The listing builds one solid part. Answer for the finished solid, in the listing's coordinates (mm). A direction names the side the tool comes from. Round coordinates to 2 decimals unless told otherwise and drop trailing zeros. Write each loop counter-clockwise with the first axis right and the second up, starting at its lowest first coordinate (ties: lowest second). Pieces come first, ordered by that corner, then holes. Notation, with made-up numbers: M -16,34 L 22,34 A14 ccw 22,46 Z; hole C 65,16.25 d1. An arc over 180 degrees is marked long. Answer as CSV lines item,"result". Start each with the question number.
from build123d import *

# Parameters (mm, degrees)
SKETCH_1_R               = 70
EXTRUDE_1_DEPTH          = 12
SKETCH_2_R               = 20
EXTRUDE_2_DEPTH          = 12
SKETCH_3_R               = 8
CUT_EXTRUDE_1_DEPTH      = 102.862652626
CUT_EXTRUDE_2_DEPTH      = 102.862652626
PATTERN_CIRCULAR_1_COUNT = 6
SKETCH_5_R               = 32
CUT_EXTRUDE_3_DEPTH      = 141
PATTERN_CIRCULAR_2_COUNT = 6
SKETCH_6_R               = 4
CUT_EXTRUDE_4_DEPTH      = 140.642
SKETCH_8_R               = 2.5
CUT_EXTRUDE_7_DEPTH      = 13


with BuildPart() as part:
    # Sketch 1 → Extrude 1 (new body)
    with BuildSketch(Plane.XY):
        Circle(SKETCH_1_R)
    extrude(amount=EXTRUDE_1_DEPTH)

    # Sketch 2 → Extrude 2 (add)
    with BuildSketch(Plane.XY.offset(12)):
        Circle(SKETCH_2_R)
    extrude(amount=EXTRUDE_2_DEPTH)

    # Sketch 3 → Cut-Extrude 1 (cut, through all)
    with BuildSketch(Plane.XY):
        Circle(SKETCH_3_R)
    extrude(amount=CUT_EXTRUDE_1_DEPTH, mode=Mode.SUBTRACT)

    # Sketch 4 → Cut-Extrude 2 (cut, through all)
    with BuildSketch(Plane.XY):
        with BuildLine():
            Line((75, -5), (40, -5))
            ThreePointArc((40, -5), (35, 0), (40, 5))
            Line((40, 5), (75, 5))
            Line((75, 5), (75, -5))
        make_face()
    cut_extrude_2 = extrude(amount=CUT_EXTRUDE_2_DEPTH, mode=Mode.SUBTRACT)

    # Pattern Circular 1: Cut-Extrude 2 ×6 about axis
    pattern_circular_1_axis = Axis((0, 0, 0), (0, 0, 1))
    for i in range(1, PATTERN_CIRCULAR_1_COUNT):
        add(cut_extrude_2.rotate(pattern_circular_1_axis, i * 360 / PATTERN_CIRCULAR_1_COUNT), mode=Mode.SUBTRACT)

    # Sketch 5 → Cut-Extrude 3 (cut, symmetric)
    with BuildSketch(Plane.XY):
        with Locations((69.282, 40)):
            Circle(SKETCH_5_R)
    cut_extrude_3 = extrude(amount=CUT_EXTRUDE_3_DEPTH, both=True, mode=Mode.SUBTRACT)

    # Pattern Circular 2: Cut-Extrude 3 ×6 about axis
    pattern_circular_2_axis = Axis((0, 0, 0), (0, 0, 1))
    for i in range(1, PATTERN_CIRCULAR_2_COUNT):
        add(cut_extrude_3.rotate(pattern_circular_2_axis, i * 360 / PATTERN_CIRCULAR_2_COUNT), mode=Mode.SUBTRACT)

    # Sketch 6 → Cut-Extrude 4 (cut, symmetric)
    with BuildSketch(Plane.XY):
        with Locations((24.248711, 14)):
            Circle(SKETCH_6_R)
        with Locations((0, 28)):
            Circle(SKETCH_6_R)
        with Locations((-24.248711, 14)):
            Circle(SKETCH_6_R)
        with Locations((-24.248711, -14)):
            Circle(SKETCH_6_R)
        with Locations((0, -28)):
            Circle(SKETCH_6_R)
        with Locations((24.248711, -14)):
            Circle(SKETCH_6_R)
    extrude(amount=CUT_EXTRUDE_4_DEPTH, both=True, mode=Mode.SUBTRACT)

    # Sketch 8 → Cut-Extrude 7 (cut)
    with BuildSketch(Plane(origin=(20, 0, 0), x_dir=(0, 0, -1), z_dir=(1, 0, 0))):
        with Locations((-18, 0)):
            Circle(SKETCH_8_R)
    extrude(amount=-CUT_EXTRUDE_7_DEPTH, mode=Mode.SUBTRACT)


solid = part.part
Q1. Find section C-C (z = 4.75). Count the separate pieces of the cut face and the enclosed holes in it, plus the area to 3 significant figures.
Q2. The mould has two halves that part along Y. Classify faces 1 (the face through (69.695, -6.523, 5.916)), 2 (the face through (-1.73, -7.81, 11.83)), 3 (the face through (-4.336, -19.524, 17.916)): +Y half, -Y half, draft (parallel to the pull), parting line (faces both ways), or undercut.
Q3. Find section B-B (y = -53). Determine the outline of the cut face in (x, z).
Q4. Find section D-D (y = 14). Determine the outline of the cut face in (x, z), plus the area to 3 significant figures.
Q5. Each of these flat-tipped pins is pushed along its axis until it touches: P1, Ø9.5, axis at x = 51.5, z = 4, coming from the +Y side; P2, Ø9.5, axis at x = 0, y = 0, coming from the +Z side; P3, Ø4, axis at x = 52, z = 6, coming from the +Y side; P4, Ø13, axis at x = -24.25, y = 14, coming from the +Z side. Where does it stop, or does it pass through?
Q6. Find section A-A (y = 0). Determine the outline of the cut face in (x, z), plus the area to 3 significant figures.
Q7. For faces 4 (the face through (-35, 0, 6)), 5 (the face through (-31.89, -45.235, 5.916)), determine the directions among +Z, -Z, +X, -X, +Y, -Y from which every point of the face is accessible in a straight line to the end or side of a thin tool.
Q8. Straight lines are drawn through the part: L1, parallel to Y at x = 0, z = 3.25; L2, parallel to X at y = 14, z = 8.25; L3, parallel to X at y = 33, z = 2. For each, find the intervals that lie inside material, in ascending order.
Reported:
1,separate pieces,"1"
1,enclosed holes,"7"
1,area,"7,710 mm2"
2,face 1,"-Y half"
2,face 2,"undercut"
2,face 3,"parting line"
3,outline,"M -40.04,0 L -36.37,0 L -36.37,12 L -40.04,12 Z; M -24.83,0 L -17.18,0 L -17.18,12 L -24.83,12 Z; M 17.18,0 L 24.83,0 L 24.83,12 L 17.18,12 Z; M 36.37,0 L 40.04,0 L 40.04,12 L 36.37,12 Z"
4,outline,"M -50.63,0 L -28.25,0 L -28.25,12 L -50.63,12 Z; M -20.25,0 L 20.25,0 L 20.25,12 L 14.28,12 L 14.28,24 L -14.28,24 L -14.28,12 L -20.25,12 Z; M 28.25,0 L 50.63,0 L 50.63,12 L 28.25,12 Z"
4,area,"1,370 mm2"
5,P1,"stops at y = 17.28"
5,P2,"passes through"
5,P3,"stops at y = 14.46"
5,P4,"stops at z = 12"
6,outline,"M -35,0 L -8,0 L -8,24 L -20,24 L -20,12 L -35,12 Z; M 8,0 L 35,0 L 35,12 L 20,12 L 20,15.5 L 8,15.5 Z; M 8,20.5 L 20,20.5 L 20,24 L 8,24 Z"
6,area,"876 mm2"
7,face 4,"+Z, -Z, -X"
7,face 5,"+Z, -Z"
8,L1,"y = -48 to -32, -24 to -8, 8 to 24, 32 to 48"
8,L2,"x = -50.63 to -28.25, -20.25 to 20.25, 28.25 to 50.63"
8,L3,"x = -38.06 to -24.83, -15.28 to 15.28, 24.83 to 38.06"
